```python
from build123d import *

# Parameters (mm, degrees)
SKETCH1_W           = 4.3942
SKETCH1_H           = 5.715
BOSS_EXTRUDE1_DEPTH = 0.7493
SKETCH4_W           = 0.5
SKETCH4_H           = 12.7
SKETCH4_H_2         = 13.7
BOSS_EXTRUDE2_DEPTH = 0.25


with BuildPart() as part:
    # Sketch1 → Boss-Extrude1 (new body, symmetric)
    with BuildSketch(Plane.XY):
        Rectangle(SKETCH1_W, SKETCH1_H)
    extrude(amount=BOSS_EXTRUDE1_DEPTH, both=True)

    # Sketch3 → Revolve1 (revolve)
    with BuildSketch(Plane(origin=(0, 0, 0), x_dir=(0, 0, -1), z_dir=(1, 0, 0))):
        with BuildLine():
            Line((-1.4993, 1.6375), (-0.7493, 1.6375))
            Line((-0.7493, 1.6375), (-0.7493, 2.3875))
            ThreePointArc((-0.7493, 2.3875), (-1.279630086, 2.167830086), (-1.4993, 1.6375))
        make_face()
    revolve(axis=Axis((0, 1.6375, 2.078989668), (0, 0, -1)))

    # Sketch4 → Boss-Extrude2 (add, symmetric)
    with BuildSketch(Plane.XY):
        with Locations((-1.27, -9.2075)):
            Rectangle(SKETCH4_W, SKETCH4_H)
        with Locations((1.27, -9.7075)):
            Rectangle(SKETCH4_W, SKETCH4_H_2)
    extrude(amount=BOSS_EXTRUDE2_DEPTH, both=True)


solid = part.part
```
Geometry check sheet. Reference: the model listing, model coordinates, mm. Coordinates: 2 decimals unless noted, no trailing zeros. Order: outer loops, then holes, each group sorted by start corner. A loop starts at its lowest first (then second) coordinate and runs counter-clockwise, first axis right, second up. Notation, with made-up numbers: (-5.5, 6.25) - (28.5, 6.25) arc R12 ccw to (28.5, 27.25) - close; hole circle Ø2 at (-36, 18). An arc over 180 degrees is marked (long way). Answer as a JSON object with one key per item and string values. Group by question number.
Item 1: Depth check by flat-ended pin: pin 1 Ø1.5 at (x, y) = (-0.5, -5.5) entering from -Z; pin 2 Ø0.6 at (x, z) = (-1.5, 0) entering from -Y; pin 3 Ø0.6 at (x, y) = (-1, -9) entering from +Z. Enter the tip coordinate at first touch or a pass-through.
Item 2: Sectioned sample at C-C, the plane z = -0.5. Record the cut outline in (x, y).
Item 3: Draft check along X on faces 1 (the face through (-2.197, 0, 0)), 2 (the face through (0, 0, 0.749)), 3 (the face through (2.197, 0, 0)), 4 (the face through (0, -2.858, 0)). Enter one of: +X half, -X half, draft (parallel to the pull), parting line (faces both ways), or undercut.
Item 4: Scan lines: probe 1 along Y at (x, z) = (-0.7, 0.2); probe 2 along Z at (x, y) = (0.9, 0.25); probe 3 along X at (y, z) = (-13.25, 0.1). Record each from-to range of solid material in increasing order.
Item 5: Sectioned sample at B-B, the plane x = 1.3. Record the cut outline in (y, z), and give its area (3 significant figures).
Item 6: Sectioned sample at D-D, the plane y = -0.75. Record the cut outline in (x, z).
Item 7: Sectioned sample at A-A, the plane y = -10.25. Record the cut outline in (x, z).
Resolved:
{
 "1": {"pin 1": "z = -0.25", "pin 2": "y = -15.56", "pin 3": "z = 0.25"},
 "2": {"outline": "(-2.2, -2.86) - (2.2, -2.86) - (2.2, 2.86) - (-2.2, 2.86) - close"},
 "3": {"face 1": "-X half", "face 2": "draft", "face 3": "+X half", "face 4": "undercut"},
 "4": {"probe 1": "-2.86 to 2.86", "probe 2": "-0.75 to 0.75", "probe 3": "-1.52 to -1.02, 1.02 to 1.52"},
 "5": {"outline": "(-16.56, -0.25) - (-2.86, -0.25) - (-2.86, -0.75) - (2.86, -0.75) - (2.86, 0.75) - (-2.86, 0.75) - (-2.86, 0.25) - (-16.56, 0.25) - close", "area": "15.4 mm^2"},
 "6": {"outline": "(-2.2, -0.75) - (2.2, -0.75) - (2.2, 0.75) - (-2.2, 0.75) - close"},
 "7": {"outline": "(-1.52, -0.25) - (-1.02, -0.25) - (-1.02, 0.25) - (-1.52, 0.25) - close; (1.02, -0.25) - (1.52, -0.25) - (1.52, 0.25) - (1.02, 0.25) - close"}
}
